Work out the finished part from the listing and answer in its coordinate system (mm). A direction names the side the tool comes from. Coordinates: 2 decimals unless noted, no trailing zeros. Order: outer loops, then holes, each group sorted by start corner. A loop starts at its lowest first (then second) coordinate and runs counter-clockwise, first axis right, second up. Notation, with made-up numbers: (5, -6) -> (27, -6) arc R21 cw to (27, 26) -> close; hole circle Ø2 at (61, 39.5). An arc over 180 degrees is marked (long way). Answer as CSV lines item,"result". Start each with the question number.
Item 1: Each of these flat-tipped pins is pushed along its axis until it touches: pin 1 Ø2.5 at (y, z) = (-7.5, 6) entering from -X; pin 2 Ø2.5 at (y, z) = (-4.5, 4) entering from -X; pin 3 Ø2.5 at (y, z) = (-7, -6) entering from +X; pin 4 Ø4.5 at (y, z) = (-5.5, -6) entering from -X. Where does it stop, or does it pass through?
Item 2: Section A-A (z = 0) is taken. Count the separate pieces of the cut face and the enclosed holes in it, then the cut area to 3 significant figures.
Item 3: Section D-D (y = -10.5) is taken. Write down the section's boundary in (x, z).
Item 4: Which of the six approach directions +Z, -Z, +X, -X, +Y, -Y give full straight-line access (tool end or side, diameter ignored) to faces 5 (the face through (-1, -3.5, -5)), 6 (the face through (12.7, -7.5, 5.8)), 7 (the face through (12.7, -8, -6)), 8 (the face through (10.714, 6.347, -0.05))?
Item 5: For a pull along X with two mould halves and no side action, classify faces 1 (the face through (2.32, -12.46, -5.6)), 2 (the face through (14.7, -7.5, 5.8)), 3 (the face through (-1.27, -4.01, -5.45)), 4 (the face through (5.5, 3.7, 5.1)) as pulls with the +X half, pulls with the -X half, needs draft (parallel to the pull), parting line crosses it, or undercut.
Item 6: Section B-B (x = 10) is taken. Write down the section's boundary in (y, z), then the cut area to 3 significant figures.
Item 7: Section C-C (x = 15.35) is taken. Write down the section's boundary in (y, z).
Item 8: Straight lines are drawn through the part: L1, parallel to X at y = 2.5, z = 6.5; L2, parallel to X at y = 0, z = 7; L3, parallel to Y at x = 10, z = 2.5. For each, find the intervals that lie inside material, in ascending order.
```python
from build123d import *

# Parameters (mm, degrees)
EXTRUDE_1_DEPTH          = 17.7
FILLET_1_R               = 1.5
EXTRUDE_2_DEPTH          = 2.5
EXTRUDE_2_DEPTH_BACK     = 20.2
EXTRUDE_3_DEPTH          = 1
MIRROR_6_COPY_1_DEPTH    = 1
SKETCH_5_R               = 0.6
EXTRUDE_4_DEPTH          = 6
EXTRUDE_6_DEPTH          = 1.5
SKETCH_9_R               = 7.5
CUT_EXTRUDE_1_DEPTH      = 2
PATTERN_LINEAR_1_COUNT   = 2
PATTERN_LINEAR_1_PITCH   = 3
MIRROR_8_COPY_1_SKETCH_R = 7.5
MIRROR_8_COPY_1_DEPTH    = 2


with BuildPart() as part:
    # Эскиз1 → Бобышка-Вытянуть1 (new body)
    with BuildSketch(Plane(origin=(0, 0, 0), x_dir=(0, 0, -1), z_dir=(1, 0, 0))):
        Polygon((-7.5, 2.5), (-3.5, 4.5), (-3.5, 9.5), (3.5, 9.5), (3.5, 4.5), (7.5, 2.5), (7.5, -6.5), (6, -9.5), (-6, -9.5), (-7.5, -6.5), align=None)
    extrude(amount=EXTRUDE_1_DEPTH)

    # Скругление1
    fillet_1_edges = [part.edges().sort_by_distance(p)[0] for p in [
        (8.85, 2.5, -7.5),
        (8.85, -6.5, -7.5),
        (8.85, -6.5, 7.5),
        (8.85, 2.5, 7.5),
        (8.85, 9.5, 3.5),
        (8.85, 9.5, -3.5),
    ]]
    fillet(fillet_1_edges, radius=FILLET_1_R)

    # Эскиз2 → Бобышка-Вытянуть2 (add, two sides: drawn at the far end of the back side and taken through both)
    with BuildSketch(Plane.ZY.offset(-EXTRUDE_2_DEPTH_BACK)):
        with BuildLine():
            Line((-2, 9.5), (2, 9.5))
            ThreePointArc((2, 9.5), (3.06066, 9.06066), (3.5, 8))
            Line((3.5, 8), (3.5, -4.5))
            Line((3.5, -4.5), (-3.5, -4.5))
            Line((-3.5, -4.5), (-3.5, 8))
            ThreePointArc((-3.5, 8), (-3.06066, 9.06066), (-2, 9.5))
        make_face()
    extrude(amount=EXTRUDE_2_DEPTH + EXTRUDE_2_DEPTH_BACK)

    # Эскиз4 → Бобышка-Вытянуть3 (add)
    with BuildSketch(Plane.XZ.offset(4.5)):
        Polygon((0, 3.5), (-2.5, 3.5), (0, 7.464813), align=None)
    extrude_3 = extrude(amount=-EXTRUDE_3_DEPTH)

    # Зеркальное отражение4: Бобышка-Вытянуть3 across plane
    add(extrude_3.mirror(Plane.XY))

    # Зеркальное отражение6: Бобышка-Вытянуть3 across plane
    add(extrude_3.mirror(Plane.ZY.offset(-8.85)))

    # Зеркальное отражение6 copy 1 sketch → Зеркальное отражение6 copy 1 (add)
    with BuildSketch(Plane(origin=(17.7, -4.5, 0), x_dir=(-1, 0, 0), z_dir=(0, -1, 0))):
        Polygon((0, 3.5), (-2.5, 3.5), (0, 7.464813), align=None)
    extrude(amount=-MIRROR_6_COPY_1_DEPTH)

    # Эскиз5 → Бобышка-Вытянуть4 (add)
    with BuildSketch(Plane.XZ.offset(9.5)):
        with Locations(Location((2.35, 5, 0), (0, 0, 90))):
            Circle(SKETCH_5_R)
        with Locations(Location((15.35, 5, 0), (0, 0, 90))):
            Circle(SKETCH_5_R)
        with Locations(Location((15.35, -5, 0), (0, 0, 90))):
            Circle(SKETCH_5_R)
        with Locations(Location((2.35, -5, 0), (0, 0, 90))):
            Circle(SKETCH_5_R)
    extrude(amount=EXTRUDE_4_DEPTH)

    # Эскиз8 → Бобышка-Вытянуть6 (add, symmetric)
    with BuildSketch(Plane.XY):
        Polygon((2, -9.5), (0, -9.5), (1.577317, -11.5), (2, -11.5), align=None)
    extrude_6 = extrude(amount=EXTRUDE_6_DEPTH, both=True)

    # Зеркальное отражение7: Бобышка-Вытянуть6 across plane
    add(extrude_6.mirror(Plane.ZY.offset(-8.85)))

    # Эскиз9 → Вырез-Вытянуть1 (cut)
    with BuildSketch(Plane.ZY.offset(-3)):
        with BuildLine():
            Line((-4.744729, -9.5), (-6, -9.5))
            Line((-6, -9.5), (-7.307128, -6.885745))
            ThreePointArc((-7.307128, -6.885745), (0, 6.347609), (7.307128, -6.885745))
            Line((7.307128, -6.885745), (6, -9.5))
            Line((6, -9.5), (4.744729, -9.5))
            ThreePointArc((4.744729, -9.5), (0, -10.920558), (-4.744729, -9.5))
        make_face()
        with Locations((0, -2.286475)):
            Circle(SKETCH_9_R, mode=Mode.SUBTRACT)
    cut_extrude_1 = extrude(amount=-CUT_EXTRUDE_1_DEPTH, mode=Mode.SUBTRACT)

    # Линейный массив1: Вырез-Вытянуть1 ×2
    with Locations(*[(i * PATTERN_LINEAR_1_PITCH, 0, 0) for i in range(1, PATTERN_LINEAR_1_COUNT)]):
        add(cut_extrude_1, mode=Mode.SUBTRACT)

    # Зеркальное отражение8: Вырез-Вытянуть1 across plane
    add(cut_extrude_1.mirror(Plane.ZY.offset(-8.85)), mode=Mode.SUBTRACT)

    # Зеркальное отражение8 copy 1 sketch → Зеркальное отражение8 copy 1 (cut)
    with BuildSketch(Plane(origin=(11.7, 0, 0), x_dir=(0, 0, 1), z_dir=(1, 0, 0))):
        with BuildLine():
            Line((-4.744729, 9.5), (-6, 9.5))
            Line((-6, 9.5), (-7.307128, 6.885745))
            ThreePointArc((-7.307128, 6.885745), (0, -6.347609), (7.307128, 6.885745))
            Line((7.307128, 6.885745), (6, 9.5))
            Line((6, 9.5), (4.744729, 9.5))
            ThreePointArc((4.744729, 9.5), (0, 10.920558), (-4.744729, 9.5))
        make_face()
        with Locations((0, 2.286475)):
            Circle(MIRROR_8_COPY_1_SKETCH_R, mode=Mode.SUBTRACT)
    extrude(amount=-MIRROR_8_COPY_1_DEPTH, mode=Mode.SUBTRACT)


solid = part.part
```
Checked values:
1,pin 1,"stops at x = 0"
1,pin 2,"stops at x = -2.5"
1,pin 3,"stops at x = 17.7"
1,pin 4,"stops at x = -2.19"
2,separate pieces,"1"
2,enclosed holes,"4"
2,area,"402 mm^2"
3,outline,"(0.79, -1.5) -> (2, -1.5) -> (2, 1.5) -> (0.79, 1.5) -> close; circle Ø1.2 at (2.35, -5); circle Ø1.2 at (2.35, 5); circle Ø1.2 at (15.35, -5); circle Ø1.2 at (15.35, 5); (15.7, -1.5) -> (16.91, -1.5) -> (16.91, 1.5) -> (15.7, 1.5) -> close"
4,face 5,"-Z, -X, +Y"
4,face 6,"+Z, -Y"
4,face 7,"-Z, -Y"
4,face 8,"none"
5,face 1,"undercut"
5,face 2,"undercut"
5,face 3,"pulls with the -X half"
5,face 4,"needs draft"
6,outline,"(-9.5, -2.05) arc R7.5 ccw (long way) to (-9.5, 2.05) -> close; (5.61, -3.5) -> (8, -3.5) arc R1.5 ccw to (9.5, -2) -> (9.5, 2) arc R1.5 ccw to (8, 3.5) -> (5.61, 3.5) arc R8.63 cw to start"
6,area,"199 mm^2"
7,outline,"(-15.5, -5.6) -> (-9.5, -5.6) -> (-9.5, -6) -> (-6.82, -7.34) arc R1.5 ccw to (-6.15, -7.5) -> (1.57, -7.5) arc R1.5 ccw to (2.91, -6.67) -> (4.5, -3.5) -> (8, -3.5) arc R1.5 ccw to (9.5, -2) -> (9.5, 2) arc R1.5 ccw to (8, 3.5) -> (4.5, 3.5) -> (2.91, 6.67) arc R1.5 ccw to (1.57, 7.5) -> (-6.15, 7.5) arc R1.5 ccw to (-6.82, 7.34) -> (-9.5, 6) -> (-9.5, 5.6) -> (-15.5, 5.6) -> (-15.5, 4.4) -> (-9.5, 4.4) -> (-9.5, -4.4) -> (-15.5, -4.4) -> close"
8,L1,"x = 0 to 3, 5 to 6, 8 to 9.7, 11.7 to 12.7, 14.7 to 17.7"
8,L2,"x = 0 to 17.7"
8,L3,"y = -9.36 to 4.78, 5.98 to 9.41"
